For this review, use the dimensioned drawing (mm, ordinates from the lowest corner) and the shaded views. A direction names the side the tool comes from. Coordinates: 2 decimals unless noted, no trailing zeros. Order: outer loops, then holes, each group sorted by start corner. A loop starts at its lowest first (then second) coordinate and runs counter-clockwise, first axis right, second up. Notation, with made-up numbers: (74.5, 26.25) -> (90.5, 26.25) arc R31 cw to (90.5, 63.25) -> close; hole circle Ø1 at (19, -1). An arc over 180 degrees is marked (long way). Use one line per item in the form item = value. Start each with the question number.
(1) Wall thickness on line 1 along X through (y, z) = (26.5, 36.5); line 2 along Y through (x, z) = (54.75, 45); line 3 along Z through (x, y) = (41, 6): over which ranges is each line inside the solid? List them lowest first.
(2) Take a section at A-A (x = 9). State the section outline as (y, z) points, then the cut area to 3 significant figures.
(3) Mouldability with a two-part tool opening along Y and no side actions: class the marked faces 6, 7, 8 and 9 as +Y half, -Y half, draft (parallel to the pull), parting line (faces both ways), or undercut.
(4) For the marked faces 1, 2, 3, 4 and 5, list the 3-axis set-ups (+Z, -Z, +X, -X, +Y, -Y) from which the entire face can be reached by the end or side of a thin tool; tool diameter is ignored.
(5) Take a section at B-B (y = 22). State the section outline as (x, z) points, then the cut area to 3 significant figures.
(6) Take a section at C-C (z = 48.5). State the section outline as (x, y) points (1 decimal), then the cut area to 3 significant figures.
(7) Take a section at D-D (x = 28.5). State the section outline as (y, z) points, then the cut area to 3 significant figures.
(8) Insertion check: pin 1 Ø13 at (x, z) = (55, 15) entering from -Y; pin 2 Ø12 at (x, y) = (39.5, 22.5) entering from +Z; pin 3 Ø18.5 at (x, z) = (4.5, 26.5) entering from +Y. Each pin has a flat end and moves straight along its axis. Give the tip position at first contact, or say it passes through.
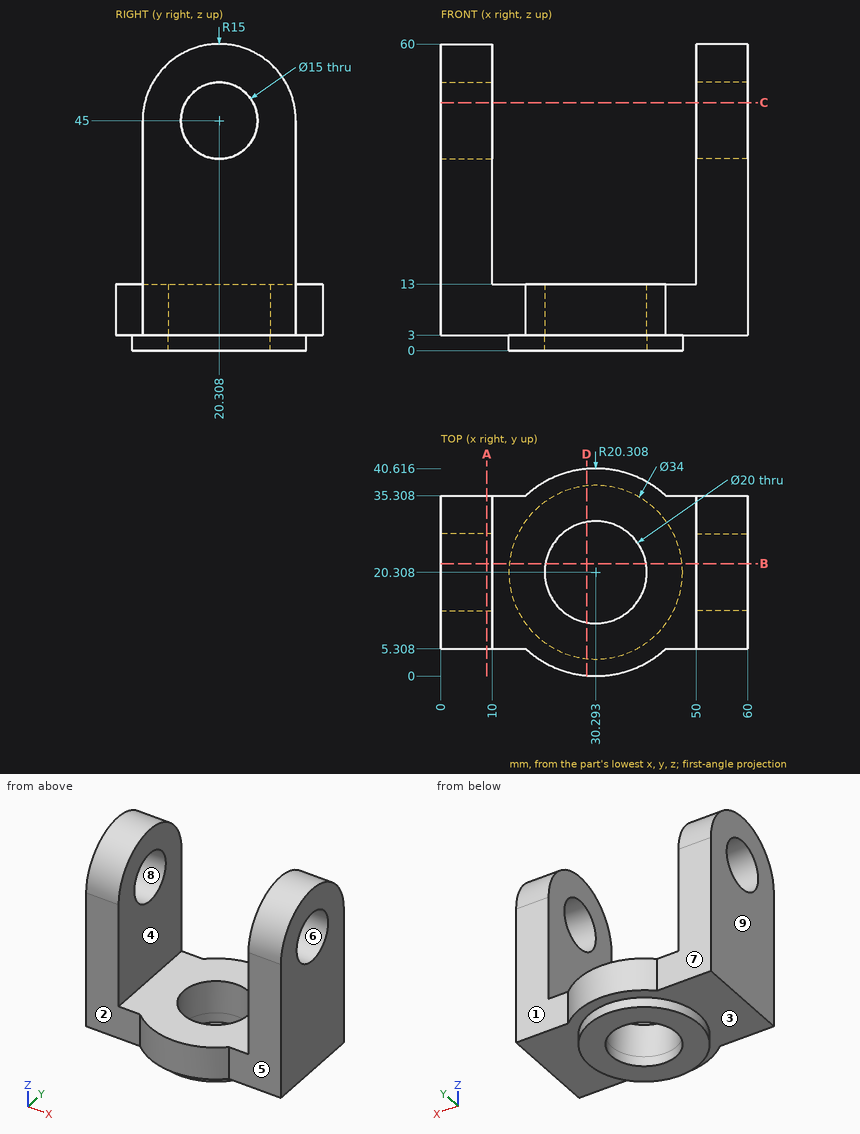
Findings:
q1.line_1 = 0 to 10, 50 to 60
q1.line_2 = 5.31 to 12.81, 27.81 to 35.31
q1.line_3 = 3 to 13
q2.outline = (5.31, 3) -> (35.31, 3) -> (35.31, 45) arc R15 ccw to (5.31, 45) -> close; hole circle Ø15 at (20.31, 45)
q2.area = 1,440 mm²
q3.face_6 = undercut
q3.face_7 = +Y half
q3.face_8 = undercut
q3.face_9 = draft
q4.face_1 = +Z, -Z, +X, +Y
q4.face_2 = +Z, -Z, -X, -Y
q4.face_3 = -Z
q4.face_4 = +Z, +Y, -Y
q4.face_5 = +Z, -Z, +X, -Y
q5.outline = (0, 3) -> (13.38, 3) -> (13.38, 0) -> (20.44, 0) -> (20.44, 13) -> (10, 13) -> (10, 37.69) -> (0, 37.69) -> close; (0, 52.31) -> (10, 52.31) -> (10, 59.9) -> (0, 59.9) -> close; (40.15, 0) -> (47.21, 0) -> (47.21, 3) -> (60, 3) -> (60, 37.69) -> (50, 37.69) -> (50, 13) -> (40.15, 13) -> close; (50, 52.31) -> (60, 52.31) -> (60, 59.9) -> (50, 59.9) -> close
q5.area = 1,090 mm²
q6.outline = (0, 5.7) -> (10, 5.7) -> (10, 13.7) -> (0, 13.7) -> close; (0, 26.9) -> (10, 26.9) -> (10, 34.9) -> (0, 34.9) -> close; (50, 5.7) -> (60, 5.7) -> (60, 13.7) -> (50, 13.7) -> close; (50, 26.9) -> (60, 26.9) -> (60, 34.9) -> (50, 34.9) -> close
q6.area = 318 mm²
q7.outline = (0.08, 3) -> (3.4, 3) -> (3.4, 0) -> (10.47, 0) -> (10.47, 13) -> (0.08, 13) -> close; (30.15, 0) -> (37.21, 0) -> (37.21, 3) -> (40.54, 3) -> (40.54, 13) -> (30.15, 13) -> close
q7.area = 250 mm²
q8.pin_1 = 5.31
q8.pin_2 = 13
q8.pin_3 = 35.31
